```python
from build123d import *

# Parameters (mm, degrees)
F0_R     = 6
F1_DEPTH = 3


with BuildPart() as f1:
    # F0 (on Front) → F1 (new body)
    with BuildSketch(Plane.XZ):
        with BuildLine():
            Line((40.156027, 16.157978), (40.156027, 28.157978))
            Line((40.156027, 28.157978), (43.156027, 28.157978))
            Line((43.156027, 28.157978), (43.156027, 40.157978))
            Line((43.156027, 40.157978), (40.156027, 40.157978))
            Line((40.156027, 40.157978), (-74.851933, 40.157978))
            ThreePointArc((-74.851933, 40.157978), (-95.337215, 48.64326), (-86.851933, 28.157978))
            Line((-86.851933, 28.157978), (-83.851933, 28.157978))
            Line((-83.851933, 28.157978), (-83.851933, 16.157978))
            Line((-83.851933, 16.157978), (-86.851933, 16.157978))
            Line((-86.851933, 16.157978), (-86.851933, 4.157978))
            Line((-86.851933, 4.157978), (-83.851933, 4.157978))
            Line((-83.851933, 4.157978), (-83.851933, -7.842022))
            Line((-83.851933, -7.842022), (-86.851933, -7.842022))
            Line((-86.851933, -7.842022), (-86.851933, -16.842022))
            Line((-86.851933, -16.842022), (-83.851933, -16.842022))
            Line((-83.851933, -16.842022), (-72.399493, -16.842022))
            Line((-72.399493, -16.842022), (-72.399493, -19.842022))
            Line((-72.399493, -19.842022), (-57.955053, -19.842022))
            Line((-57.955053, -19.842022), (-57.955053, -16.842022))
            Line((-57.955053, -16.842022), (-43.510613, -16.842022))
            Line((-43.510613, -16.842022), (-43.510613, -19.842022))
            Line((-43.510613, -19.842022), (-29.066173, -19.842022))
            Line((-29.066173, -19.842022), (-29.066173, -16.842022))
            Line((-29.066173, -16.842022), (-14.621733, -16.842022))
            Line((-14.621733, -16.842022), (-14.621733, -19.842022))
            Line((-14.621733, -19.842022), (-0.177293, -19.842022))
            Line((-0.177293, -19.842022), (-0.177293, -16.842022))
            Line((-0.177293, -16.842022), (14.267147, -16.842022))
            Line((14.267147, -16.842022), (14.267147, -19.842022))
            Line((14.267147, -19.842022), (28.711587, -19.842022))
            Line((28.711587, -19.842022), (28.711587, -16.842022))
            Line((28.711587, -16.842022), (40.156027, -16.842022))
            Line((40.156027, -16.842022), (43.156027, -16.842022))
            Line((43.156027, -16.842022), (43.156027, -7.842022))
            Line((43.156027, -7.842022), (40.156027, -7.842022))
            Line((40.156027, -7.842022), (40.156027, 4.157978))
            Line((40.156027, 4.157978), (43.156027, 4.157978))
            Line((43.156027, 4.157978), (43.156027, 16.157978))
            Line((43.156027, 16.157978), (40.156027, 16.157978))
        make_face()
        with Locations((-86.851933, 40.157978)):
            Circle(F0_R, mode=Mode.SUBTRACT)
    extrude(amount=F1_DEPTH)


solid = f1.part
```
Source: CAD feature listing. Evaluate the final solid. Frame: model axes, mm. A direction names the side the tool comes from. Round coordinates to 2 decimals unless told otherwise and drop trailing zeros. Loops run counter-clockwise (first coordinate to the right, second up) from the corner with the lowest first, then second, coordinate; pieces in that order, holes last. Notation, with made-up numbers: M -21,-12 L -9,-12 A30 ccw -9,19 Z; hole C 26,65 d10. An arc over 180 degrees is marked long. Use a Markdown table: item, result. Add a question column.
1. Cut plane B-B, the plane x = -38. Output: boundary loops of the cut face in (y, z).
2. Ray query, line 1 along X through (y, z) = (-1.3, 11.5); line 2 along Z through (x, y) = (-39.5, -1.85); line 3 along X through (y, z) = (-2.6, -4). Return the intervals inside material, ascending. Write a range as [from, to].
3. Contact query for flat-ended pins moving along their axis: pin 1 (0.9 mm diameter, centred on y = -1, z = -18.5, fed in from +X); pin 2 (4 mm diameter, centred on x = -11, z = 4.5, fed in from +Y); pin 3 (1.5 mm diameter, centred on x = 41, y = -1, fed in from +Z); pin 4 (1.5 mm diameter, centred on y = -1, z = -1.5, fed in from -X). Output: stop coordinate, or through.
4. Set-up query: faces 1 (the flat face through (28.712, -1, -18)), 2 (the flat face through (-57.955, -1, -18)), 3 (the flat face through (-85, -1, -7.842)), 4 (the flat face through (42, -1, -7.842)). Return all of +Z, -Z, +X, -X, +Y, -Y with unobstructed straight access to the full face (end or side cutting, diameter ignored); none if empty.
5. Pull-direction query (Z, two-part tool) for faces 5 (the flat face through (40.156, -1, 22)), 6 (the flat face through (-29, 0, 9)), 7 (the flat face through (-36, -1, -19.842)); classes: +Z half, -Z half, draft (parallel to the pull), parting line (faces both ways), or undercut.
6. Cut plane A-A, the plane z = 24.5. Output: boundary loops of the cut face in (x, y), and give its area (3 significant figures).
Solution:
| question | item | result |
|---|---|---|
| 1 | outline | M -3,-19.84 L 0,-19.84 L 0,40.16 L -3,40.16 Z |
| 2 | line 1 | x = [-86.85, 43.16] |
| 2 | line 2 | z = [-19.84, 40.16] |
| 2 | line 3 | x = [-83.85, 40.16] |
| 3 | pin 1 | stops at x = 28.71 |
| 3 | pin 2 | stops at y = 0 |
| 3 | pin 3 | stops at z = 40.16 |
| 3 | pin 4 | stops at x = -83.85 |
| 4 | face 1 | -Z, +X, +Y, -Y |
| 4 | face 2 | -Z, +Y, -Y |
| 4 | face 3 | -X, +Y, -Y |
| 4 | face 4 | +X, +Y, -Y |
| 5 | face 5 | undercut |
| 5 | face 6 | draft |
| 5 | face 7 | -Z half |
| 6 | outline | M -83.85,-3 L 40.16,-3 L 40.16,0 L -83.85,0 Z |
| 6 | area | 372 mm2 |
